```python
from build123d import *

# Parameters (mm, degrees)
SKETCH3_W           = 180
SKETCH3_H           = 180
BOSS_EXTRUDE1_DEPTH = 3.18
CUT_EXTRUDE1_DEPTH  = 128.318939675
SKETCH5_R           = 1.436023081
SKETCH5_W           = 3.18
SKETCH5_H           = 80.125
CUT_EXTRUDE2_DEPTH  = 128.318939675


with BuildPart() as part:
    # Sketch3 → Boss-Extrude1 (new body)
    with BuildSketch(Plane.XY):
        Rectangle(SKETCH3_W, SKETCH3_H)
        Polygon((44.679729843, -65), (-5.320270157, -65), (-5.320270157, 65), (44.679729843, 65), (44.679729843, 10.125), (47.859729843, 10.125), (47.859729843, 1.5), (51.859729843, 1.5), (51.859729843, 3.5), (54.859729843, 3.5), (54.859729843, 1.5), (57.679729843, 1.5), (57.679729843, -1.5), (54.859729843, -1.5), (54.859729843, -3.5), (51.859729843, -3.5), (51.859729843, -1.5), (47.859729843, -1.5), (47.859729843, -9.875), (44.679729843, -9.875), align=None, mode=Mode.SUBTRACT)
    extrude(amount=BOSS_EXTRUDE1_DEPTH)

    # Sketch4 → Cut-Extrude1 (cut, through all)
    with BuildSketch(Plane.XY.offset(3.18)):
        Polygon((1.5, 86.82), (10, 86.82), (10, 90), (-10, 90), (-10, 86.82), (-1.5, 86.82), (-1.5, 82.82), (-3.5, 82.82), (-3.5, 79.82), (-1.5, 79.82), (-1.5, 77), (1.5, 77), (1.5, 79.82), (3.5, 79.82), (3.5, 82.82), (1.5, 82.82), align=None)
        Polygon((1.5, -79.82), (1.5, -77), (-1.5, -77), (-1.5, -79.82), (-3.5, -79.82), (-3.5, -82.82), (-1.5, -82.82), (-1.5, -86.82), (-10, -86.82), (-10, -90), (10, -90), (10, -86.82), (1.5, -86.82), (1.5, -82.82), (3.5, -82.82), (3.5, -79.82), align=None)
    extrude(amount=-CUT_EXTRUDE1_DEPTH, mode=Mode.SUBTRACT)

    # Sketch5 → Cut-Extrude2 (cut, through all)
    with BuildSketch(Plane.XY.offset(3.18)):
        with Locations((-88, 0)):
            Circle(SKETCH5_R)
        with Locations((88, 0)):
            Circle(SKETCH5_R)
        with Locations((-88.41, 49.9375)):
            Rectangle(SKETCH5_W, SKETCH5_H)
        with Locations((-88.41, -49.9375)):
            Rectangle(SKETCH5_W, SKETCH5_H)
        with Locations((88.41, -49.9375)):
            Rectangle(SKETCH5_W, SKETCH5_H)
        with Locations((88.41, 49.9375)):
            Rectangle(SKETCH5_W, SKETCH5_H)
    extrude(amount=-CUT_EXTRUDE2_DEPTH, mode=Mode.SUBTRACT)


solid = part.part
```
Geometry check sheet. Reference: the model listing, model coordinates, mm. Give positions to 0.01 mm unless a question says otherwise; leave off trailing zeros. Order: outer loops, then holes, each group sorted by start corner. A loop starts at its lowest first (then second) coordinate and runs counter-clockwise, first axis right, second up. Notation, with made-up numbers: (-13.75, 62) - (39.25, 62) arc R34 ccw to (39.25, 96) - close; hole circle Ø9 at (49, 62). An arc over 180 degrees is marked (long way). Answer in a Markdown table with one row per item. Add a question column.
Q1. Cross-section at B-B, the plane z = 2.2. Count the separate pieces of the cut face and the enclosed holes in it, then the cut area to 3 significant figures.
Q2. Material ranges on probe 1 along Y at (x, z) = (11, 1.1); probe 2 along X at (y, z) = (-79.5, 1.7); probe 3 along Y at (x, z) = (88, 1) (3 decimals), recorded low to high. Write a range as from..to.
Q3. Cross-section at C-C, the plane y = 68.5. Enter the section's corners in (x, z), then the cut area to 3 significant figures.
Q4. Cross-section at A-A, the plane y = -27.5. Enter the section's corners in (x, z).
Q5. Gauge pin test, flat ends, axial feed: pin 1 (1 mm diameter, centred on x = -3, z = 1, fed in from +Y); pin 2 (1 mm diameter, centred on x = -3, z = 1, fed in from -Y); pin 3 (1 mm diameter, centred on y = 84, z = 1.5, fed in from -X); pin 4 (10 mm diameter, centred on x = -53.5, y = 37.5, fed in from -Z). Record the tip position at first contact, or that the pin passes through.
Check values:
| question | item | result |
|---|---|---|
| 1 | separate pieces | 1 |
| 1 | enclosed holes | 3 |
| 1 | area | 24,600 mm^2 |
| 2 | probe 1 | y = -90..-65, 65..90 |
| 2 | probe 2 | x = -86.82..-1.5, 1.5..86.82 |
| 2 | probe 3 | y = -9.875..-1.436, 1.436..9.875 |
| 3 | outline | (-86.82, 0) - (86.82, 0) - (86.82, 3.18) - (-86.82, 3.18) - close |
| 3 | area | 552 mm^2 |
| 4 | outline | (-86.82, 0) - (-5.32, 0) - (-5.32, 3.18) - (-86.82, 3.18) - close; (44.68, 0) - (86.82, 0) - (86.82, 3.18) - (44.68, 3.18) - close |
| 5 | pin 1 | stops at y = 86.82 |
| 5 | pin 2 | stops at y = -86.82 |
| 5 | pin 3 | stops at x = -86.82 |
| 5 | pin 4 | stops at z = 0 |
